The model under review builds one solid part; all positions refer to its coordinate system, in mm. A direction names the side the tool comes from. Round coordinates to 2 decimals unless told otherwise and drop trailing zeros. Order: outer loops, then holes, each group sorted by start corner. A loop starts at its lowest first (then second) coordinate and runs counter-clockwise, first axis right, second up.
```python
from build123d import *

# Parameters (mm, degrees)
SALIENTE_EXTRUIR1_DEPTH = 3
CROQUIS2_R              = 1.5
CORTAR_EXTRUIR1_DEPTH   = 141.829538188
CROQUIS3_R              = 2
CORTAR_EXTRUIR2_DEPTH   = 141.829538188


with BuildPart() as part:
    # Croquis1 → Saliente-Extruir1 (new body)
    with BuildSketch(Plane.XY):
        Polygon((-99.558924327, -2.052657564), (-68.947342436, -71.850238602), (2.052657564, -99.558924327), (71.850238602, -68.947342436), (99.558924327, 2.052657564), (68.947342436, 71.850238602), (-2.052657564, 99.558924327), (-71.850238602, 68.947342436), align=None)
    extrude(amount=SALIENTE_EXTRUIR1_DEPTH)

    # Croquis2 → Cortar-Extruir1 (cut, through all)
    with BuildSketch(Plane.XY.offset(3)):
        with Locations((6.374524738, 69.970461156)):
            Circle(CROQUIS2_R)
        with Locations(Location((42.705814706, 55.791696428, 0), (0, 0, 180))):
            Circle(CROQUIS2_R)
        with Locations((-6.374524738, -69.970461156)):
            Circle(CROQUIS2_R)
        with Locations(Location((-42.705814706, -55.791696428, 0), (0, 0, 180))):
            Circle(CROQUIS2_R)
        with Locations((-69.970461156, 6.374524738)):
            Circle(CROQUIS2_R)
        with Locations(Location((-55.791696428, 42.705814706, 0), (0, 0, 180))):
            Circle(CROQUIS2_R)
        Polygon((-67.635138809, -1.394468454), (-46.839227198, -48.811303398), (1.394468454, -67.635138809), (48.811303398, -46.839227198), (67.635138809, 1.394468454), (46.839227198, 48.811303398), (-1.394468454, 67.635138809), (-48.811303398, 46.839227198), align=None)
    extrude(amount=-CORTAR_EXTRUIR1_DEPTH, mode=Mode.SUBTRACT)

    # Croquis3 → Cortar-Extruir2 (cut, through all)
    with BuildSketch(Plane.XY.offset(3)):
        with Locations((-1.887752493, 91.560624112)):
            Circle(CROQUIS3_R)
        with Locations((63.40829561, 66.077980789)):
            Circle(CROQUIS3_R)
        with Locations((1.887752493, -91.560624112)):
            Circle(CROQUIS3_R)
        with Locations((-63.40829561, -66.077980789)):
            Circle(CROQUIS3_R)
        with Locations((-91.560624112, -1.887752493)):
            Circle(CROQUIS3_R)
        with Locations((-66.077980789, 63.40829561)):
            Circle(CROQUIS3_R)
    extrude(amount=-CORTAR_EXTRUIR2_DEPTH, mode=Mode.SUBTRACT)


solid = part.part
```
(1) Consider section B-B (z = 1.4). State how many separate pieces and enclosed holes the cut face has, and give its area (3 significant figures).
Data:
separate pieces: 1
enclosed holes: 13
area: 15,000 mm2
(2) Consider section A-A (y = 30.5). Write out the cut boundary in (x, z), and give its area (3 significant figures).
Data:
outline: (-86.85, 0) - (-55.19, 0) - (-55.19, 3) - (-86.85, 3) - close; (54.87, 0) - (87.08, 0) - (87.08, 3) - (54.87, 3) - close
area: 192 mm2
(3) Consider section D-D (x = 84.5). Write out the cut boundary in (y, z), and give its area (3 significant figures).
Data:
outline: (-36.53, 0) - (36.39, 0) - (36.39, 3) - (-36.53, 3) - close
area: 219 mm2
(4) For faces 5 (the flat face through (-84.47, -36.46, 1.48)), 6 (the flat face through (57.383, 24.771, 1.521)), list the 3-axis set-ups (+Z, -Z, +X, -X, +Y, -Y) from which the entire face can be reached by the end or side of a thin tool; tool diameter is ignored.
Data:
face 5: +Z, -Z, -X, -Y
face 6: +Z, -Z
(5) Insertion check: pin 1 (4 mm diameter, centred on x = 42.71, y = 55.79, fed in from +Z); pin 2 (1 mm diameter, centred on x = -14.5, z = 1, fed in from +Y); pin 3 (1.8 mm diameter, centred on x = -55.79, y = 42.71, fed in from -Z). Each pin has a flat end and moves straight along its axis. Give the tip position at first contact, or say it passes through.
Data:
pin 1: stops at z = 3
pin 2: stops at y = 94.32
pin 3: passes through
(6) To check wall thickness, follow probe 1 along X at (y, z) = (22.5, 2.7); probe 2 along Y at (x, z) = (44, 2.6); probe 3 along Y at (x, z) = (36, 2.8). State the ranges of each line that lie inside material, in increasing order.
Data:
probe 1: x = -89.98 to -58.31, 58.38 to 90.59
probe 2: y = -81.16 to -48.95, 49.92 to 55.03, 56.55 to 81.59
probe 3: y = -84.67 to -52.46, 53.04 to 84.71
(7) Draft analysis for pull direction Y (two halves, no side actions). For faces 1 (the flat face through (36.46, -84.47, 1.48)), 2 (the flat face through (-68, 1, 3)), 3 (the flat face through (-23.06, -58.09, 1.52)), 4 (the flat face through (-36.46, 84.47, 1.48)), state which applies: pulls with the +Y half, pulls with the -Y half, needs draft (parallel to the pull), parting line crosses it, or undercut.
Data:
face 1: pulls with the -Y half
face 2: needs draft
face 3: undercut
face 4: pulls with the +Y half
(8) Consider section C-C (x = -19). Write out the cut boundary in (y, z).
Data:
outline: (-91.34, 0) - (-59.68, 0) - (-59.68, 3) - (-91.34, 3) - close; (59.91, 0) - (92.13, 0) - (92.13, 3) - (59.91, 3) - close
